```python
from build123d import *

# Parameters (mm, degrees)
SKETCH1_R                = 50.8
BOSS_EXTRUDE1_DEPTH      = 1030
BOSS_EXTRUDE1_DEPTH_BACK = 680
SKETCH2_R                = 455
BOSS_EXTRUDE2_DEPTH      = 20
BOSS_EXTRUDE3_START      = -280
SKETCH7_R                = 305
BOSS_EXTRUDE3_DEPTH      = 620
SKETCH8_R                = 225
BOSS_EXTRUDE4_DEPTH      = 50


with BuildPart() as part:
    # Sketch1 → Boss-Extrude1 (new body, two sides)
    with BuildSketch(Plane.XY) as boss_extrude1_sk:
        Circle(SKETCH1_R)
    extrude(amount=BOSS_EXTRUDE1_DEPTH)
    extrude(boss_extrude1_sk.sketch, amount=-BOSS_EXTRUDE1_DEPTH_BACK)

    # Sketch2 → Boss-Extrude2 (add)
    with BuildSketch(Plane.XY.offset(-680)):
        Circle(SKETCH2_R)
    extrude(amount=BOSS_EXTRUDE2_DEPTH)

    # Sketch7 → Boss-Extrude3 (add)
    with BuildSketch(Plane.XY.offset(1030).offset(BOSS_EXTRUDE3_START)):
        Circle(SKETCH7_R)
    extrude(amount=-BOSS_EXTRUDE3_DEPTH)

    # Sketch8 → Boss-Extrude4 (add)
    with BuildSketch(Plane(origin=(0, 0, 130), x_dir=(-1, 0, 0), z_dir=(0, 0, -1))):
        Circle(SKETCH8_R)
    extrude(amount=BOSS_EXTRUDE4_DEPTH)


solid = part.part
```
Verification items for the finished model (mm, model axes). A direction names the side the tool comes from. Give positions to 0.01 mm unless a question says otherwise; leave off trailing zeros. Order: outer loops, then holes, each group sorted by start corner. A loop starts at its lowest first (then second) coordinate and runs counter-clockwise, first axis right, second up. Notation, with made-up numbers: M -3.75,81.5 L 10.25,81.5 A14 ccw 10.25,99.5 Z; hole C 81.25,48.25 d4. An arc over 180 degrees is marked long. Return JSON: item names as keys, results as strings. Group by question number.
1) Access from +Z, -Z, +X, -X, +Y, -Y to the whole of each face (thin tool, end or side, straight path). Record for faces 1 (the face through (433.99, 136.67, -670.14)), 2 (the face through (-304.705, 13.41, 444.34)), 3 (the face through (-11.012, -49.592, -284.82)).
2) Go/stop test with flat-tipped pins: pin 1 Ø6 at (x, z) = (268.5, 696.5) entering from +Y; pin 2 Ø1.5 at (x, y) = (171, 33) entering from +Z; pin 3 Ø10 at (x, y) = (262.5, 270) entering from +Z. Record where each tip stops, or that it passes through.
3) Scan lines: line 1 (Z direction, x = 79, y = -222); line 2 (Z direction, x = 136.5, y = 139); line 3 (Z direction, x = 15, y = 339). Record each from-to range of solid material in increasing order.
4) Section check D-D on z = -485. Record the cut outline in (x, y).
5) Section check A-A on y = 0. Record the cut outline in (x, z), and give its area (3 significant figures).
6) Section check B-B on y = -138.5. Record the cut outline in (x, z).
Answer block:
{
 "1": {"face 1": "+Z, -Z", "face 2": "+Z", "face 3": "none"},
 "2": {"pin 1": "stops at y = 150.12", "pin 2": "stops at z = 750", "pin 3": "stops at z = -660"},
 "3": {"line 1": "z = -680 to -660, 130 to 750", "line 2": "z = -680 to -660, 80 to 750", "line 3": "z = -680 to -660"},
 "4": {"outline": "C 0,0 d101.6"},
 "5": {"outline": "M -455,-680 L 455,-680 L 455,-660 L 50.8,-660 L 50.8,80 L 225,80 L 225,130 L 305,130 L 305,750 L 50.8,750 L 50.8,1030 L -50.8,1030 L -50.8,750 L -305,750 L -305,130 L -225,130 L -225,80 L -50.8,80 L -50.8,-660 L -455,-660 Z", "area": "523,000 mm^2"},
 "6": {"outline": "M -433.41,-680 L 433.41,-680 L 433.41,-660 L -433.41,-660 Z; M -271.74,130 L -177.32,130 L -177.32,80 L 177.32,80 L 177.32,130 L 271.74,130 L 271.74,750 L -271.74,750 Z"}
}
